Can you work these out from the drawing? Everything is in mm from the part's minimum corner. Coordinates: 2 decimals unless noted, no trailing zeros. Write each loop counter-clockwise with the first axis right and the second up, starting at its lowest first coordinate (ties: lowest second). Pieces come first, ordered by that corner, then holes. Notation, with made-up numbers: (45.5, -20) -> (82.5, -20) arc R20 cw to (82.5, -13) -> close; hole circle Ø6 at (56.25, 54.5). An arc over 180 degrees is marked (long way). Use a Markdown table: item, result. Add a question column.
Item 1: Imagine slicing it at D-D, the plane y = 8.75. Write out the boundary of the cut face in (x, z), and give its area (3 significant figures).
Item 2: If I drill on line 1 along X through (y, z) = (2.05, 6.5) (1 decimal); line 2 along Z through (x, y) = (6.5, 3.15); line 3 along X through (y, z) = (5.55, 6.5) (1 decimal), over which ranges is the centre line in solid material (lowest first)? Write a range as from..to.
Item 3: Imagine slicing it at A-A, the plane z = 6.5. Write out the boundary of the cut face in (x, y) (1 decimal), and give its area (3 significant figures).
Item 4: Imagine slicing it at B-B, the plane y = 2.75. Write out the boundary of the cut face in (x, z).
Item 5: Imagine slicing it at C-C, the plane x = 75. Write out the boundary of the cut face in (y, z).
Item 6: If we mould it in two halves opening along Y, with no side actions, what happens to the marked faces 1, 2 and 3? For each: pulls with the +Y half, pulls with the -Y half, needs draft (parallel to the pull), parting line crosses it, or undercut.
Item 7: Will these pins go through, and if not, where does the flat tip stop? pin 1 Ø5 at (x, z) = (6.5, 6.5) entering from -Y; pin 2 Ø2 at (y, z) = (2.5, 22) entering from +X; pin 3 Ø2.5 at (x, z) = (7.5, 7.5) entering from +Y; pin 4 Ø14.5 at (x, z) = (6.5, 6.5) entering from +Y.
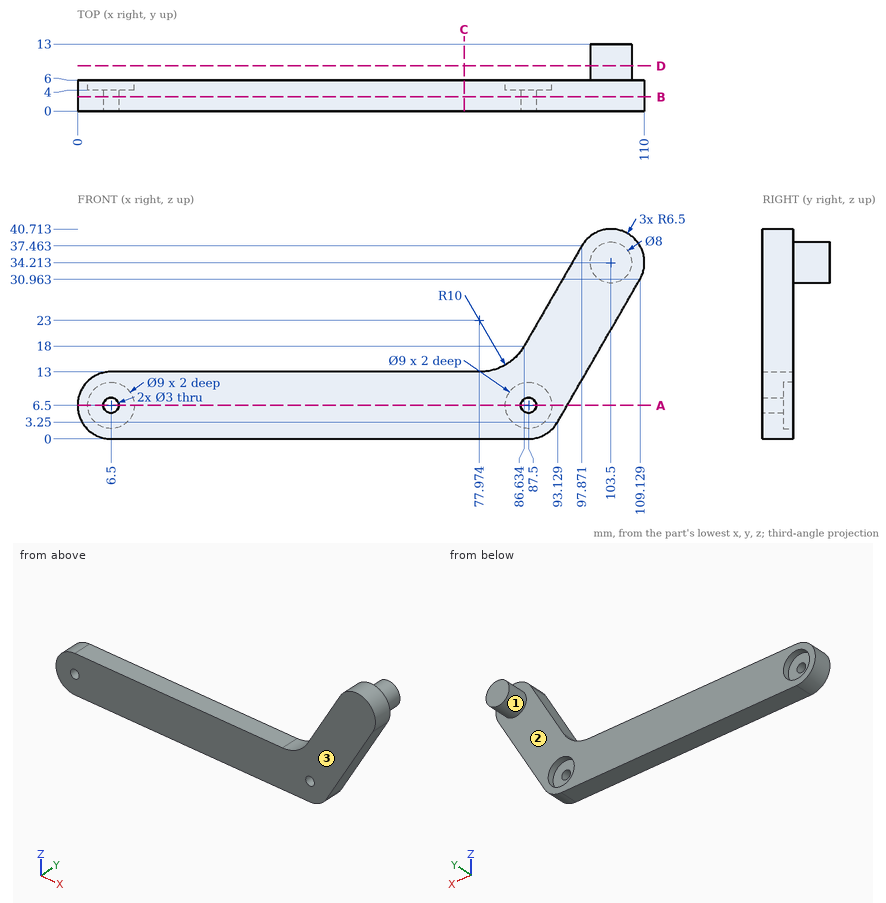
Ans:
| question | item | result |
|---|---|---|
| 1 | outline | circle Ø8 at (103.5, 34.21) |
| 1 | area | 50.3 mm^2 |
| 2 | line 1 | x = 0..5, 8..86, 89..95 |
| 2 | line 2 | z = 0..5, 8..13 |
| 2 | line 3 | x = 0..2, 11..83, 92..95 |
| 3 | outline | (0, 0) -> (5, 0) -> (5, 4) -> (2, 4) -> (2, 6) -> (0, 6) -> close; (8, 0) -> (86, 0) -> (86, 4) -> (83, 4) -> (83, 6) -> (11, 6) -> (11, 4) -> (8, 4) -> close; (89, 0) -> (95, 0) -> (95, 6) -> (92, 6) -> (92, 4) -> (89, 4) -> close |
| 3 | area | 510 mm^2 |
| 4 | outline | (6.5, 0) -> (87.5, 0) arc R6.5 ccw to (93.13, 3.25) -> (109.13, 30.96) arc R6.5 ccw to (97.87, 37.46) -> (86.63, 18) arc R10 cw to (77.97, 13) -> (6.5, 13) arc R6.5 ccw to start; hole circle Ø3 at (6.5, 6.5); hole circle Ø3 at (87.5, 6.5) |
| 5 | outline | (0, 0) -> (6, 0) -> (6, 13) -> (0, 13) -> close |
| 6 | face 1 | needs draft |
| 6 | face 2 | pulls with the +Y half |
| 6 | face 3 | pulls with the -Y half |
| 7 | pin 1 | stops at y = 0 |
| 7 | pin 2 | stops at x = 104.53 |
| 7 | pin 3 | stops at y = 4 |
| 7 | pin 4 | stops at y = 6 |
